Verification items for this drawing (mm, ordinates from the low corner). A direction names the side the tool comes from. Coordinates: 2 decimals unless noted, no trailing zeros. Loops run counter-clockwise (first coordinate to the right, second up) from the corner with the lowest first, then second, coordinate; pieces in that order, holes last. Notation, with made-up numbers: M 67.5,31.5 L 93.5,31.5 A15 cw 93.5,56.5 Z; hole C 24,63.25 d6. An arc over 180 degrees is marked long. Return JSON: item names as keys, results as strings.
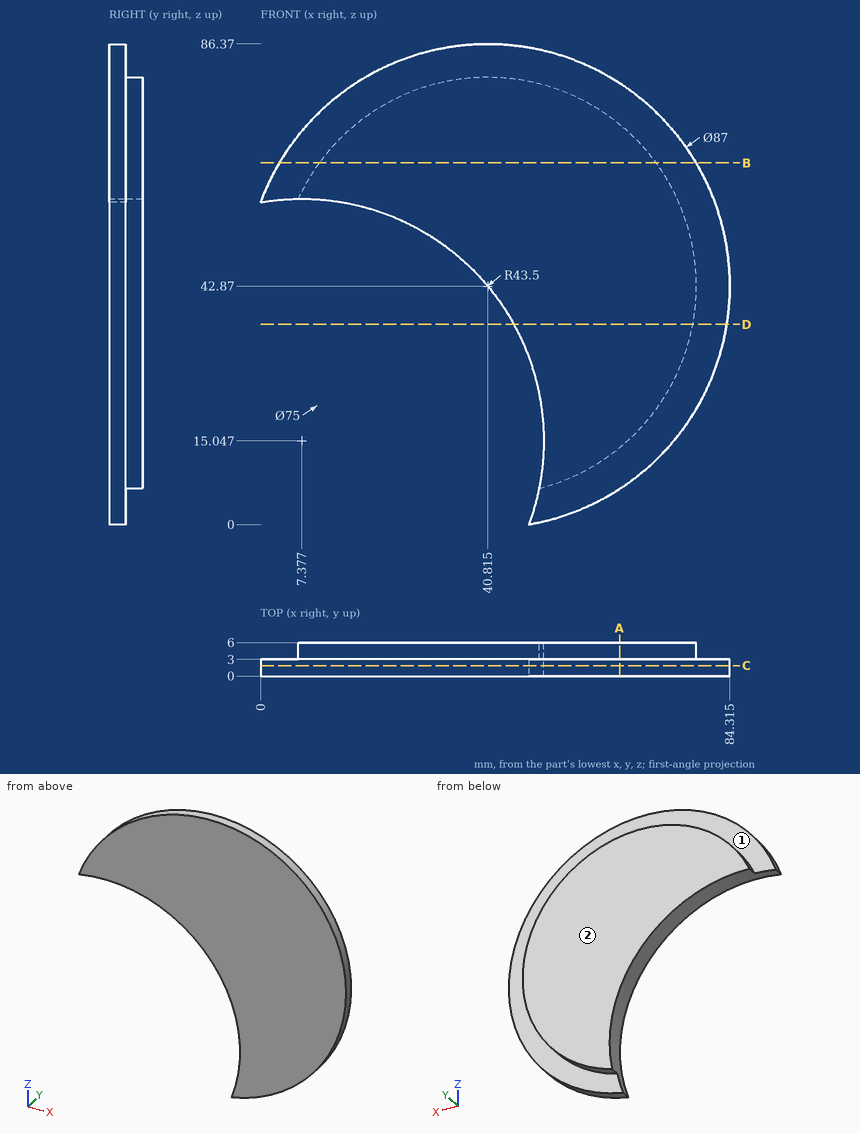
1) Section check B-B on z = 65. Record the cut outline in (x, y) (1 decimal).
Answers:
{"outline": "M 3.4,0 L 78.3,0 L 78.3,3 L 71.1,3 L 71.1,6 L 10.5,6 L 10.5,3 L 3.4,3 Z"}
2) Section check D-D on z = 36. Record the cut outline in (x, y), then the cut area to 3 significant figures.
Answers:
{"outline": "M 45.5,0 L 83.77,0 L 83.77,3 L 77.68,3 L 77.68,6 L 45.5,6 Z", "area": "211 mm²"}
3) Scan lines: line 1 along X through (y, z) = (3.35, 40) (1 decimal); line 2 along Z through (x, y) = (20.5, 5.2); line 3 along Z through (x, y) = (66.5, 1.15). Record each from-to range of solid material in increasing order. Write a range as [from, to].
Answers:
{"line 1": "[43, 78.2]", "line 2": "[56.52, 74.39]", "line 3": "[7.76, 77.98]"}
4) Section check C-C on y = 1.85. Record the cut outline in (x, z) (1 decimal), then the cut area to 3 significant figures.
Answers:
{"outline": "M 0,57.9 A43.5 cw 48.2,0 A43.5 ccw long Z", "area": "3,620 mm²"}
5) Set-up check for the marked faces 1 and 2: record each of +Z, -Z, +X, -X, +Y, -Y from which the full face is reachable in a straight line by a thin tool's end or side.
Answers:
{"face 1": "+Y", "face 2": "+Z, -Z, +X, -X, +Y"}
6) Go/stop test with flat-tipped pins: pin 1 Ø3 at (y, z) = (4.5, 36) entering from -X; pin 2 Ø1 at (x, y) = (35.5, 4.5) entering from -Z; pin 3 Ø1.5 at (y, z) = (4.5, 13) entering from -X. Record where each tip stops, or that it passes through.
Answers:
{"pin 1": "x = 44.63", "pin 2": "z = 47.8", "pin 3": "x = 50.79"}
7) Section check A-A on x = 64.5. Record the cut outline in (y, z).
Answers:
{"outline": "M 0,6.38 L 3,6.38 L 3,13.8 L 6,13.8 L 6,71.94 L 3,71.94 L 3,79.36 L 0,79.36 Z"}
